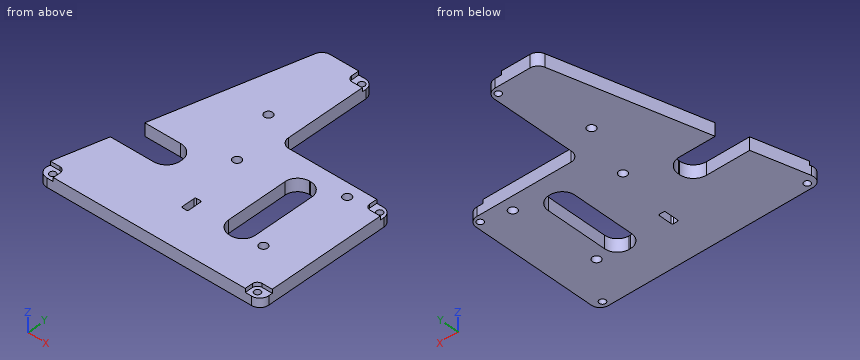
```python
from build123d import *

# Parameters (mm, degrees)
BOSS_EXTRUDE1_DEPTH = 10
CUT_EXTRUDE1_DEPTH  = 10
SKETCH3_R           = 3.25
CUT_EXTRUDE2_DEPTH  = 10
CUT_EXTRUDE3_DEPTH  = 3
SKETCH5_R           = 2.5
CUT_EXTRUDE4_DEPTH  = 7


with BuildPart() as part:
    # Sketch1 → Boss-Extrude1 (new body)
    with BuildSketch(Plane.XY):
        with BuildLine():
            Line((89.21038961, -16.914285714), (15.21038961, -16.914285714))
            ThreePointArc((15.21038961, -16.914285714), (10.260642142, -14.864033183), (8.21038961, -9.914285714))
            Line((8.21038961, -9.914285714), (8.21038961, 56.085714286))
            ThreePointArc((8.21038961, 56.085714286), (6.160137079, 61.035461754), (1.21038961, 63.085714286))
            Line((1.21038961, 63.085714286), (-26.351704849, 63.085714286))
            ThreePointArc((-26.351704849, 63.085714286), (-30.646070949, 61.613681345), (-33.134308946, 57.816691373))
            Line((-33.134308946, 57.816691373), (-78.561392279, -120.183308627))
            ThreePointArc((-78.561392279, -120.183308627), (-77.306755242, -126.208651814), (-71.778788183, -128.914285714))
            Line((-71.778788183, -128.914285714), (89.21038961, -128.914285714))
            ThreePointArc((89.21038961, -128.914285714), (94.160137079, -126.864033183), (96.21038961, -121.914285714))
            Line((96.21038961, -121.914285714), (96.21038961, -23.914285714))
            ThreePointArc((96.21038961, -23.914285714), (94.160137079, -18.964538246), (89.21038961, -16.914285714))
        make_face()
    extrude(amount=BOSS_EXTRUDE1_DEPTH)

    # Sketch2 → Cut-Extrude1 (cut)
    with BuildSketch(Plane.XY.offset(10)):
        with BuildLine():
            Line((-68.029193723, -55.914285714), (-34.029193723, -55.914285714))
            ThreePointArc((-34.029193723, -55.914285714), (-26.25101913, -59.136111121), (-23.029193723, -66.914285714))
            Line((-23.029193723, -66.914285714), (-23.029193723, -67.914285714))
            ThreePointArc((-23.029193723, -67.914285714), (-26.25101913, -75.692460307), (-34.029193723, -78.914285714))
            Line((-34.029193723, -78.914285714), (-68.029193723, -78.914285714))
            Line((-68.029193723, -78.914285714), (-68.029193723, -55.914285714))
        make_face()
    extrude(amount=-CUT_EXTRUDE1_DEPTH, mode=Mode.SUBTRACT)

    # Sketch3 → Cut-Extrude2 (cut)
    with BuildSketch(Plane.XY.offset(10)):
        with Locations((-14.78961039, -1.914285714)):
            Circle(SKETCH3_R)
        with Locations((0.21038961, -44.914285714)):
            Circle(SKETCH3_R)
        with Locations((70.21038961, -26.914285714)):
            Circle(SKETCH3_R)
        with Locations((65.21038961, -92.914285714)):
            Circle(SKETCH3_R)
        with BuildLine():
            Line((7.21038961, -86.914285714), (10.21038961, -86.914285714))
            ThreePointArc((10.21038961, -86.914285714), (10.917496392, -87.207178933), (11.21038961, -87.914285714))
            Line((11.21038961, -87.914285714), (11.21038961, -97.914285714))
            ThreePointArc((11.21038961, -97.914285714), (10.917496392, -98.621392495), (10.21038961, -98.914285714))
            Line((10.21038961, -98.914285714), (7.21038961, -98.914285714))
            ThreePointArc((7.21038961, -98.914285714), (6.503282829, -98.621392495), (6.21038961, -97.914285714))
            Line((6.21038961, -97.914285714), (6.21038961, -87.914285714))
            ThreePointArc((6.21038961, -87.914285714), (6.503282829, -87.207178933), (7.21038961, -86.914285714))
        make_face()
        with BuildLine():
            Line((44.21038961, -30.914285714), (45.21038961, -30.914285714))
            ThreePointArc((45.21038961, -30.914285714), (52.281457422, -33.843217902), (55.21038961, -40.914285714))
            Line((55.21038961, -40.914285714), (55.21038961, -88.914285714))
            ThreePointArc((55.21038961, -88.914285714), (52.281457422, -95.985353526), (45.21038961, -98.914285714))
            Line((45.21038961, -98.914285714), (44.21038961, -98.914285714))
            ThreePointArc((44.21038961, -98.914285714), (37.139321799, -95.985353526), (34.21038961, -88.914285714))
            Line((34.21038961, -88.914285714), (34.21038961, -40.914285714))
            ThreePointArc((34.21038961, -40.914285714), (37.139321799, -33.843217902), (44.21038961, -30.914285714))
        make_face()
    extrude(amount=-CUT_EXTRUDE2_DEPTH, mode=Mode.SUBTRACT)

    # Sketch4 → Cut-Extrude3 (cut)
    with BuildSketch(Plane.XY.offset(10)):
        with BuildLine():
            Line((96.21038961, -118.914285714), (88.21038961, -118.914285714))
            ThreePointArc((88.21038961, -118.914285714), (85.381962486, -120.08585859), (84.21038961, -122.914285714))
            Line((84.21038961, -122.914285714), (84.21038961, -128.914285714))
            Line((84.21038961, -128.914285714), (96.21038961, -128.914285714))
            Line((96.21038961, -128.914285714), (96.21038961, -118.914285714))
        make_face()
        with BuildLine():
            Line((-66.778788183, -128.914285714), (-78.778788183, -128.914285714))
            Line((-78.778788183, -128.914285714), (-78.778788183, -118.914285714))
            Line((-78.778788183, -118.914285714), (-70.778788183, -118.914285714))
            ThreePointArc((-70.778788183, -118.914285714), (-67.950361058, -120.08585859), (-66.778788183, -122.914285714))
            Line((-66.778788183, -122.914285714), (-66.778788183, -128.914285714))
        make_face()
        with BuildLine():
            Line((84.21038961, -16.914285714), (96.21038961, -16.914285714))
            Line((96.21038961, -16.914285714), (96.21038961, -26.914285714))
            Line((96.21038961, -26.914285714), (88.21038961, -26.914285714))
            ThreePointArc((88.21038961, -26.914285714), (85.381962486, -25.742712839), (84.21038961, -22.914285714))
            Line((84.21038961, -22.914285714), (84.21038961, -16.914285714))
        make_face()
        with BuildLine():
            Line((-3.78961039, 63.085714286), (8.21038961, 63.085714286))
            Line((8.21038961, 63.085714286), (8.21038961, 53.085714286))
            Line((8.21038961, 53.085714286), (0.21038961, 53.085714286))
            ThreePointArc((0.21038961, 53.085714286), (-2.618037514, 54.257287161), (-3.78961039, 57.085714286))
            Line((-3.78961039, 57.085714286), (-3.78961039, 63.085714286))
        make_face()
    extrude(amount=-CUT_EXTRUDE3_DEPTH, mode=Mode.SUBTRACT)

    # Sketch5 → Cut-Extrude4 (cut)
    with BuildSketch(Plane.XY.offset(7)):
        with Locations((-71.778788183, -123.914285714)):
            Circle(SKETCH5_R)
        with Locations((89.21038961, -123.914285714)):
            Circle(SKETCH5_R)
        with Locations((91.21038961, -21.914285714)):
            Circle(SKETCH5_R)
        with Locations((3.21038961, 58.085714286)):
            Circle(SKETCH5_R)
    extrude(amount=-CUT_EXTRUDE4_DEPTH, mode=Mode.SUBTRACT)


solid = part.part
```
CAD build for the part. Positions are in the model's coordinates, mm. Round coordinates to 2 decimals unless told otherwise and drop trailing zeros. Order: outer loops, then holes, each group sorted by start corner. A loop starts at its lowest first (then second) coordinate and runs counter-clockwise, first axis right, second up. Notation, with made-up numbers: (6, 49.5) -> (17, 49.5) arc R19 ccw to (17, 73.5) -> close; hole circle Ø7 at (30, -9). An arc over 180 degrees is marked (long way). One line per question, with ' | ' between items.
Q1. Slice it at D-D (z = 4.75). Give the number of separate pieces and of enclosed holes in the cut face, then the cut area to 3 significant figures.
Completed:
separate pieces: 1 | enclosed holes: 10 | area: 19,700 mm^2
Q2. Probe probe 1 along X at (y, z) = (-88.5, 4.5); probe 2 along X at (y, z) = (-47, 1.5); probe 3 along Y at (x, z) = (2.5, 5.5). List the from-to ranges inside material, lowest first.
Completed:
probe 1: x = -70.48 to 6.21, 11.21 to 34.21, 55.21 to 96.21 | probe 2: x = -59.88 to -2.28, 2.7 to 34.21, 55.21 to 96.21 | probe 3: y = -128.91 to -47.22, -42.61 to 55.69, 60.48 to 62.97
Q3. Slice it at C-C (x = 21.5). Write the cut outline in (y, z), then the cut area to 3 significant figures.
Completed:
outline: (-128.91, 0) -> (-16.91, 0) -> (-16.91, 10) -> (-128.91, 10) -> close | area: 1,120 mm^2
Q4. Slice it at B-B (y = -74). Write the cut outline in (x, z).
Completed:
outline: (-24.87, 0) -> (34.21, 0) -> (34.21, 10) -> (-24.87, 10) -> close; (55.21, 0) -> (96.21, 0) -> (96.21, 10) -> (55.21, 10) -> close
Q5. Drop flat-ended pins along their axis: pin 1 (8 mm diameter, centred on x = 91.21, y = -21.91, fed in from +Z); pin 2 (3.5 mm diameter, centred on x = 92.5, z = 8.5, fed in from -Y); pin 3 (5 mm diameter, centred on y = -72, z = 3.5, fed in from -X); pin 4 (6 mm diameter, centred on x = 0.21, y = -44.91, fed in from +Z). Give the stop position or say it passes through.
Completed:
pin 1: stops at z = 7 | pin 2: stops at y = -128.49 | pin 3: stops at x = -25.22 | pin 4: passes through
Q6. Slice it at A-A (x = 40). Write the cut outline in (y, z).
Completed:
outline: (-128.91, 0) -> (-97.98, 0) -> (-97.98, 10) -> (-128.91, 10) -> close; (-31.84, 0) -> (-16.91, 0) -> (-16.91, 10) -> (-31.84, 10) -> close
